from build123d import *

# Parameters (mm, degrees)
F1_DEPTH = 30
F3_DEPTH = 5
F4_R     = 4
F5_DEPTH = 15
F6_R     = 6
F7_DEPTH = 20


with BuildPart() as f1:
    # F0 (on Top) → F1 (new body)
    with BuildSketch(Plane.XY):
        with BuildLine():
            ThreePointArc((7, 2), (5.535534, 5.535534), (2, 7))
            Line((2, 7), (-2, 7))
            ThreePointArc((-2, 7), (-5.535534, 5.535534), (-7, 2))
            Line((-7, 2), (-7, -2))
            ThreePointArc((-7, -2), (-5.535534, -5.535534), (-2, -7))
            Line((-2, -7), (2, -7))
            ThreePointArc((2, -7), (5.535534, -5.535534), (7, -2))
            Line((7, -2), (7, 2))
        make_face()
    extrude(amount=F1_DEPTH)

    # F2 (on face) → F3 (join)
    with BuildSketch(Plane.XY.offset(30)):
        with BuildLine():
            ThreePointArc((5.7, 3.1), (4.938478, 4.938478), (3.1, 5.7))
            Line((3.1, 5.7), (-3.1, 5.7))
            ThreePointArc((-3.1, 5.7), (-4.938478, 4.938478), (-5.7, 3.1))
            Line((-5.7, 3.1), (-5.7, -3.1))
            ThreePointArc((-5.7, -3.1), (-4.938478, -4.938478), (-3.1, -5.7))
            Line((-3.1, -5.7), (3.1, -5.7))
            ThreePointArc((3.1, -5.7), (4.938478, -4.938478), (5.7, -3.1))
            Line((5.7, -3.1), (5.7, 3.1))
        make_face()
    extrude(amount=F3_DEPTH)

    # F4 (on face) → F5 (cut)
    with BuildSketch(Plane.XY.offset(35)):
        Circle(F4_R)
    extrude(amount=-F5_DEPTH, mode=Mode.SUBTRACT)

    # F6 (on face) → F7 (cut)
    with BuildSketch(Plane(origin=(0, 0, 0), x_dir=(1, 0, 0), z_dir=(0, 0, -1))):
        Circle(F6_R)
    extrude(amount=-F7_DEPTH, mode=Mode.SUBTRACT)


solid = f1.part
Design review of the part built by this model. Coordinates are the model's own, in mm. A direction names the side the tool comes from. Coordinates: 2 decimals unless noted, no trailing zeros. Write each loop counter-clockwise with the first axis right and the second up, starting at its lowest first coordinate (ties: lowest second). Pieces come first, ordered by that corner, then holes. Notation, with made-up numbers: (83, 35) - (138, 35) arc R17 ccw to (138, 48) - close; hole circle Ø8 at (86.25, 83). An arc over 180 degrees is marked (long way). One line per item, written item: value.
1) Add section A-A (z = 21). State the section outline as (x, y) points, plus the area to 3 significant figures.
Answer sheet:
outline: (-7, -2) arc R5 ccw to (-2, -7) - (2, -7) arc R5 ccw to (7, -2) - (7, 2) arc R5 ccw to (2, 7) - (-2, 7) arc R5 ccw to (-7, 2) - close; hole circle Ø8 at (0, 0)
area: 124 mm2
2) Add section D-D (z = 6). State the section outline as (x, y) points, plus the area to 3 significant figures.
Answer sheet:
outline: (-7, -2) arc R5 ccw to (-2, -7) - (2, -7) arc R5 ccw to (7, -2) - (7, 2) arc R5 ccw to (2, 7) - (-2, 7) arc R5 ccw to (-7, 2) - close; hole circle Ø12 at (0, 0)
area: 61.4 mm2
3) Insertion check: pin 1 (4 mm diameter, centred on y = 5.5, z = 24, fed in from +X); pin 2 (2.5 mm diameter, centred on x = 0.5, z = 33, fed in from -Y); pin 3 (2.5 mm diameter, centred on x = 0.5, z = 33, fed in from +Y). Each pin has a flat end and moves straight along its axis. Give the tip position at first contact, or say it passes through.
Answer sheet:
pin 1: stops at x = 6.77
pin 2: stops at y = -5.7
pin 3: stops at y = 5.7
4) For faces 1 (the face through (0, -5.7, 32)), 2 (the face through (0, 5.7, 32)), 3 (the face through (4.959, 4.918, 32.465)), 4 (the face through (4.918, -4.959, 32.465)), 5 (the face through (-6, 1, 30)), list the 3-axis set-ups (+Z, -Z, +X, -X, +Y, -Y) from which the entire face can be reached by the end or side of a thin tool; tool diameter is ignored.
Answer sheet:
face 1: +Z, +X, -X, -Y
face 2: +Z, +X, -X, +Y
face 3: +Z, +X, +Y
face 4: +Z, +X, -Y
face 5: +Z
5) Add section B-B (x = 0). State the section outline as (y, z) points.
Answer sheet:
outline: (-7, 0) - (-6, 0) - (-6, 20) - (-4, 20) - (-4, 35) - (-5.7, 35) - (-5.7, 30) - (-7, 30) - close; (4, 20) - (6, 20) - (6, 0) - (7, 0) - (7, 30) - (5.7, 30) - (5.7, 35) - (4, 35) - close
6) To check wall thickness, follow probe 1 along Y at (x, z) = (0, 32.5); probe 2 along Y at (x, z) = (0, 28); probe 3 along X at (y, z) = (0, 9). State the ranges of each line that lie inside material, in increasing order.
Answer sheet:
probe 1: y = -5.7 to -4, 4 to 5.7
probe 2: y = -7 to -4, 4 to 7
probe 3: x = -7 to -6, 6 to 7
7) Mouldability with a two-part tool opening along Y and no side actions: class faces 6 (the face through (-6, 0, 10)), 7 (the face through (5, -6, 15)), 8 (the face through (-4, 3, 35)) as +Y half, -Y half, draft (parallel to the pull), parting line (faces both ways), or undercut.
Answer sheet:
face 6: undercut
face 7: -Y half
face 8: draft
